Drawing for the job (mm, zero at the part's lowest x, y, z). A direction names the side the tool comes from. Coordinates: 2 decimals unless noted, no trailing zeros. Loops run counter-clockwise (first coordinate to the right, second up) from the corner with the lowest first, then second, coordinate; pieces in that order, holes last. Notation, with made-up numbers: (-9, 37) -> (22, 37) arc R31 cw to (22, 67) -> close; hole circle Ø1 at (59, 36). An arc over 180 degrees is marked (long way). Write item = value, one per line. Start each with the question number.
(1) Flat gauge pins, fed straight in: P1, Ø1.5, axis at x = 45, y = 7.5, coming from the +Z side; P2, Ø4, axis at y = 14.5, z = 47, coming from the +X side; P3, Ø17.5, axis at x = 30, z = 38, coming from the -Y side; P4, Ø5, axis at y = 2.5, z = 59.5, coming from the -X side. Where does each tip first touch, or does it go through?
(2) Pull direction X, two halves, no side cores. Call the marked faces 3, 4 and 5: +X half, -X half, draft (parallel to the pull), parting line (faces both ways), or undercut.
(3) Tool access for the marked faces 1 and 2: list every direction of +Z, -Z, +X, -X, +Y, -Y with a clear straight run to the whole face (end or side of a thin tool).
(4) Drill centre lines: line 1 (Z direction, x = 30, y = 9); line 2 (X direction, y = 6, z = 3); line 3 (X direction, y = 3.75, z = 28). Where is each one in solid material? Low to high. Write a range as from..to.
(5) Band-saw the part on A-A (x = 30). Write the cut outline in (y, z), and give its area (4 significant figures).
(6) Band-saw the part on D-D (x = 17). Write the cut outline in (y, z), and give its area (3 significant figures).
(7) Band-saw the part on B-B (z = 8). Write the cut outline in (x, y).
(8) Band-saw the part on C-C (y = 13.5). Write the cut outline in (x, z).
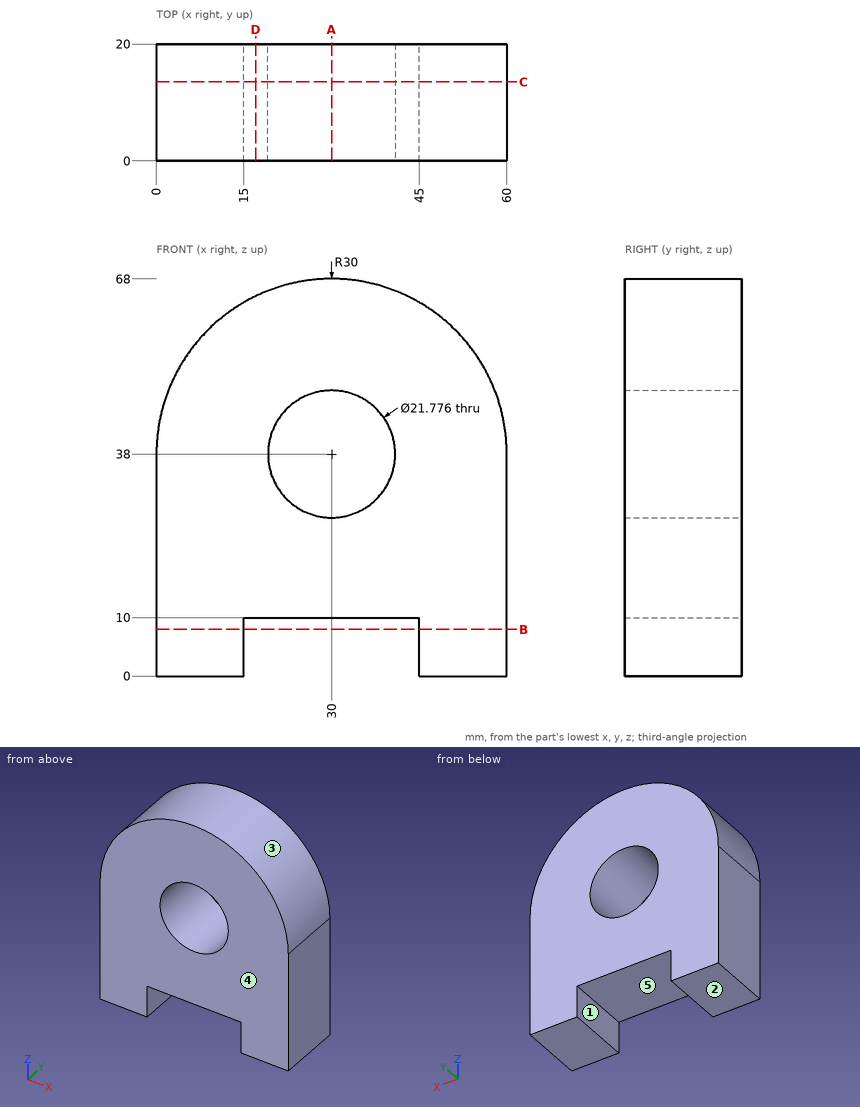
Findings below:
q1.P1 = 64.4
q1.P2 = 59.17
q1.P3 = through
q1.P4 = 6.78
q2.face_3 = parting line
q2.face_4 = draft
q2.face_5 = undercut
q3.face_1 = -Z, +Y, -Y
q3.face_2 = -Z, +X, -X, +Y, -Y
q4.line_1 = 10..27.11, 48.89..68
q4.line_2 = 0..15, 45..60
q4.line_3 = 0..25.69, 34.31..60
q5.outline = (0, 10) -> (20, 10) -> (20, 27.11) -> (0, 27.11) -> close; (0, 48.89) -> (20, 48.89) -> (20, 68) -> (0, 68) -> close
q5.area = 724.5 mm²
q6.outline = (0, 10) -> (20, 10) -> (20, 65.04) -> (0, 65.04) -> close
q6.area = 1,100 mm²
q7.outline = (0, 0) -> (15, 0) -> (15, 20) -> (0, 20) -> close; (45, 0) -> (60, 0) -> (60, 20) -> (45, 20) -> close
q8.outline = (0, 0) -> (15, 0) -> (15, 10) -> (45, 10) -> (45, 0) -> (60, 0) -> (60, 38) arc R30 ccw to (0, 38) -> close; hole circle Ø21.78 at (30, 38)
